The listing builds one solid part. Answer for the finished solid, in the listing's coordinates (mm). Round coordinates to 2 decimals unless told otherwise and drop trailing zeros. Loops run counter-clockwise (first coordinate to the right, second up) from the corner with the lowest first, then second, coordinate; pieces in that order, holes last. Notation, with made-up numbers: (56, 88.25) -> (76, 88.25) arc R11 cw to (76, 100.25) -> close; hole circle Ø1 at (-11.5, 14.25). An arc over 180 degrees is marked (long way). Write each question's results on one line, items separated by ' | '. Start each with the question number.
(1) The part is cut by section A-A (z = -34). Determine the outline of the cut face in (x, y) (3 decimals).
(2) The part is cut by section B-B (x = 14). Determine the outline of the cut face in (y, z) (3 decimals).
(3) Straight lines are drawn through the part: probe 1 along X at (y, z) = (0.45, 42.2); probe 2 along Z at (x, y) = (17, 0.5); probe 3 along X at (y, z) = (0.9, -8). For each, find the intervals that lie inside material, in ascending order.
(4) A flat-ended cylindrical pin translates along its axis: pin 1 (0.8 mm diameter, centred on y = 1, z = 15.5, fed in from -X). Find the tip coordinate at first contact, or state that the pin passes through.
(5) The part is cut by section C-C (z = 42.2). Determine the outline of the cut face in (x, y) (3 decimals).
(6) Determine the mould class of faces 1 (the face through (-39.2, 0.78, 41.84)), 2 (the face through (-43.4, 0.78, 46.43)), 3 (the face through (-43.43, 0.78, -46.4)), 4 (the face through (41.38, 0.78, -42.62)) for opening direction Z: released by +Z, released by -Z, zero draft, split by the parting line, or undercut.
(7) The part is cut by section D-D (z = -43.5). Determine the outline of the cut face in (x, y) (3 decimals).
```python
from build123d import *

# Parameters (mm, degrees)
SKETCH1_2_R         = 1.6383
SKETCH1_2_R_2       = 0.8382
BOSS_EXTRUDE2_DEPTH = 1.575
SKETCH2_W           = 14.080651801
SKETCH2_H           = 7.11628052
SKETCH2_W_2         = 15.007196354
SKETCH2_H_2         = 9.421332762
CUT_EXTRUDE1_DEPTH  = 65.400942629


with BuildPart() as part:
    # Sketch1_2 → Boss-Extrude2 (new body)
    with BuildSketch(Plane(origin=(0, 0, 0), x_dir=(1, 0, 0), z_dir=(0, 1, 0))):
        with BuildLine():
            Line((-38.39500299, 29.999999735), (-42.73000299, 29.999999735))
            Line((-42.73000299, 29.999999735), (-43.011025994, 30.003097626))
            ThreePointArc((-43.011025994, 30.003097626), (-43.710996344, 30.299838092), (-44.000003042, 31.003036872))
            Line((-44.000003042, 31.003036872), (-44.000003042, 31.269999735))
            Line((-44.000003042, 31.269999735), (-44.000005679, 44.999999735))
            ThreePointArc((-44.000005679, 44.999999735), (-43.414218633, 46.414215608), (-42.000002924, 47.000003051))
            Line((-42.000002924, 47.000003051), (-30.435003, 47.000003051))
            Line((-30.435003, 47.000003051), (-30.435003, 22.255357341))
            Line((-30.435003, 22.255357341), (-11.909003, 22.255357341))
            Line((-11.909003, 22.255357341), (-11.909003, -8.5))
            Line((-11.909003, -8.5), (-23.409003, -8.5))
            Line((-23.409003, -8.5), (-23.409003, -31.499996949))
            Line((-23.409003, -31.499996949), (23.408997, -31.499996949))
            Line((23.408997, -31.499996949), (23.408997, -8.499997555))
            Line((23.408997, -8.499997555), (11.97084713, -8.499997555))
            Line((11.97084713, -8.499997555), (11.97084713, 22.255357341))
            Line((11.97084713, 22.255357341), (30.434997, 22.255357341))
            Line((30.434997, 22.255357341), (30.434997, 47.000003051))
            Line((30.434997, 47.000003051), (42.000008541, 47.000003051))
            ThreePointArc((42.000008541, 47.000003051), (43.414213215, 46.414220704), (43.999996956, 45.000016607))
            Line((43.999996956, 45.000016607), (43.999996956, 32.000003378))
            Line((43.999996956, 32.000003378), (43.999996956, 31.015615364))
            ThreePointArc((43.999996956, 31.015615364), (43.706534093, 30.307939396), (42.998386406, 30.015616661))
            Line((42.998386406, 30.015616661), (33.825607551, 30.030389905))
            ThreePointArc((33.825607551, 30.030389905), (33.117459864, 29.738067169), (32.823997, 29.030391202))
            Line((32.823997, 29.030391202), (32.823997, -30.453996949))
            ThreePointArc((32.823997, -30.453996949), (33.116890219, -31.16110373), (33.823997, -31.453996949))
            Line((33.823997, -31.453996949), (36.099999555, -31.453996949))
            Line((36.099999555, -31.453996949), (42.849728118, -31.453996949))
            ThreePointArc((42.849728118, -31.453996949), (43.556834899, -31.746890168), (43.849728118, -32.453996949))
            Line((43.849728118, -32.453996949), (43.849728118, -36.999996949))
            Line((43.849728118, -36.999996949), (43.849728118, -46.999996949))
            Line((43.849728118, -46.999996949), (-42.000000178, -46.999996949))
            ThreePointArc((-42.000000178, -46.999996949), (-43.414212804, -46.414211581), (-44.000000499, -44.999999921))
            Line((-44.000000499, -44.999999921), (-44.000000178, -38.976999921))
            Line((-44.000000178, -38.976999921), (-44.000000178, -32.453999802))
            ThreePointArc((-44.000000178, -32.453999802), (-43.70710696, -31.746893021), (-43.000000178, -31.453999802))
            Line((-43.000000178, -31.453999802), (-36.100000549, -31.453999802))
            Line((-36.100000549, -31.453999802), (-33.824003042, -31.453999802))
            ThreePointArc((-33.824003042, -31.453999802), (-33.116896261, -31.161106583), (-32.824003042, -30.453999802))
            Line((-32.824003042, -30.453999802), (-32.824003042, 29.011483943))
            ThreePointArc((-32.824003042, 29.011483943), (-33.117785331, 29.719478678), (-33.826516131, 30.011480785))
            Line((-33.826516131, 30.011480785), (-38.39500299, 29.999999735))
        make_face()
        with Locations(Location((40, 43.5, 0), (0, 0, 270))):
            Circle(SKETCH1_2_R, mode=Mode.SUBTRACT)
        with Locations(Location((-40, 43.5, 0), (0, 0, 270))):
            Circle(SKETCH1_2_R, mode=Mode.SUBTRACT)
        with Locations(Location((-37.6, -42.2, 0), (0, 0, 270))):
            Circle(SKETCH1_2_R, mode=Mode.SUBTRACT)
        with Locations(Location((36.1, -42.2, 0), (0, 0, 270))):
            Circle(SKETCH1_2_R, mode=Mode.SUBTRACT)
        with Locations(Location((-36.785003, 36.350003051, 0), (0, 0, 270))):
            Circle(SKETCH1_2_R_2, mode=Mode.SUBTRACT)
        with Locations(Location((-26.220003, 17.93193176, 0), (0, 0, 270))):
            Circle(SKETCH1_2_R_2, mode=Mode.SUBTRACT)
        with Locations(Location((26.219997, 17.93193176, 0), (0, 0, 270))):
            Circle(SKETCH1_2_R_2, mode=Mode.SUBTRACT)
        with Locations(Location((36.784997, 36.368003051, 0), (0, 0, 270))):
            Circle(SKETCH1_2_R_2, mode=Mode.SUBTRACT)
    extrude(amount=BOSS_EXTRUDE2_DEPTH)

    # Sketch2 → Cut-Extrude1 (cut, through all)
    with BuildSketch(Plane(origin=(0, 1.575, 0), x_dir=(1, 0, 0), z_dir=(0, 1, 0))):
        with Locations((39.863054019, -29.135856689)):
            Rectangle(SKETCH2_W, SKETCH2_H)
        with Locations((-40.336598676, -27.983330568)):
            Rectangle(SKETCH2_W_2, SKETCH2_H_2)
    extrude(amount=-CUT_EXTRUDE1_DEPTH, mode=Mode.SUBTRACT)


solid = part.part
```
Checked values:
1) outline: (-44, 0) -> (-30.435, 0) -> (-30.435, 1.575) -> (-44, 1.575) -> close; (30.435, 0) -> (44, 0) -> (44, 1.575) -> (30.435, 1.575) -> close
2) outline: (0, -22.255) -> (1.575, -22.255) -> (1.575, 8.5) -> (0, 8.5) -> close; (0, 31.5) -> (1.575, 31.5) -> (1.575, 47) -> (0, 47) -> close
3) probe 1: x = -44 to -39.24, -35.96 to 34.46, 37.74 to 43.85 | probe 2: z = -22.26 to 8.5, 31.5 to 47 | probe 3: x = -32.82 to -11.91, 11.97 to 32.82
4) pin 1: stops at x = -32.82
5) outline: (-44, 0) -> (-39.238, 0) -> (-39.238, 1.575) -> (-44, 1.575) -> close; (-35.962, 0) -> (34.462, 0) -> (34.462, 1.575) -> (-35.962, 1.575) -> close; (37.738, 0) -> (43.85, 0) -> (43.85, 1.575) -> (37.738, 1.575) -> close
6) face 1: undercut | face 2: released by +Z | face 3: released by -Z | face 4: undercut
7) outline: (-44, 0) -> (-41.638, 0) -> (-41.638, 1.575) -> (-44, 1.575) -> close; (-38.362, 0) -> (-30.435, 0) -> (-30.435, 1.575) -> (-38.362, 1.575) -> close; (30.435, 0) -> (38.362, 0) -> (38.362, 1.575) -> (30.435, 1.575) -> close; (41.638, 0) -> (44, 0) -> (44, 1.575) -> (41.638, 1.575) -> close
